from build123d import *

# Parameters (mm, degrees)
SKETCH_1_W           = 50
SKETCH_1_H           = 50
EXTRUDE_1_DEPTH      = 10
SKETCH_6_R           = 10.1
CUT_EXTRUDE_4_DEPTH  = 2
SKETCH_7_R           = 5
CUT_EXTRUDE_5_DEPTH  = 72.161787499
SKETCH_10_R          = 1
CUT_EXTRUDE_6_DEPTH  = 2
SKETCH_11_R          = 1.25
CUT_EXTRUDE_7_DEPTH  = 8
SKETCH_12_R          = 1.4
CUT_EXTRUDE_8_DEPTH  = 5
FILLET_1_R           = 0.5
SKETCH_13_R          = 1.25
CUT_EXTRUDE_9_DEPTH  = 5
SKETCH_14_R          = 1.25
CUT_EXTRUDE_11_DEPTH = 6
CUT_EXTRUDE_START    = -6
SKETCH_15_R          = 1.25
CUT_EXTRUDE_12_DEPTH = 6
SKETCH_16_R          = 1.25
CUT_EXTRUDE_13_DEPTH = 6
SKETCH_17_R          = 1.25
CUT_EXTRUDE_14_DEPTH = 6


with BuildPart() as part:
    # 草图1 → 凸台-拉伸1 (new body)
    with BuildSketch(Plane(origin=(0, 0, 0), x_dir=(1, 0, 0), z_dir=(0, 1, 0))):
        with Locations((25, 25)):
            Rectangle(SKETCH_1_W, SKETCH_1_H)
    extrude(amount=EXTRUDE_1_DEPTH)

    # 草图6 → 切除-拉伸4 (cut)
    with BuildSketch(Plane(origin=(0, 0, 0), x_dir=(-1, 0, 0), z_dir=(0, -1, 0))):
        with Locations(Location((-25, 11.5, 0), (0, 0, 90))):
            Circle(SKETCH_6_R)
    extrude(amount=-CUT_EXTRUDE_4_DEPTH, mode=Mode.SUBTRACT)

    # 草图7 → 切除-拉伸5 (cut, through all)
    with BuildSketch(Plane(origin=(0, 2, 0), x_dir=(-1, 0, 0), z_dir=(0, -1, 0))):
        with Locations(Location((-25, 11.5, 0), (0, 0, 90))):
            Circle(SKETCH_7_R)
    extrude(amount=-CUT_EXTRUDE_5_DEPTH, mode=Mode.SUBTRACT)

    # 草图10 → 切除-拉伸6 (cut)
    with BuildSketch(Plane(origin=(0, 10, 0), x_dir=(1, 0, 0), z_dir=(0, 1, 0))):
        with Locations(Location((25, 39, 0), (0, 0, 270))):
            Circle(SKETCH_10_R)
        with Locations(Location((11, 11, 0), (0, 0, 270))):
            Circle(SKETCH_10_R)
        with Locations(Location((39, 11, 0), (0, 0, 270))):
            Circle(SKETCH_10_R)
    extrude(amount=-CUT_EXTRUDE_6_DEPTH, mode=Mode.SUBTRACT)

    # 草图11 → 切除-拉伸7 (cut)
    with BuildSketch(Plane(origin=(0, 0, 0), x_dir=(-1, 0, 0), z_dir=(0, -1, 0))):
        with Locations(Location((-40, 18.4, 0), (0, 0, 90))):
            Circle(SKETCH_11_R)
        with Locations(Location((-40, 4.6, 0), (0, 0, 90))):
            Circle(SKETCH_11_R)
        with Locations(Location((-10, 18.4, 0), (0, 0, 90))):
            Circle(SKETCH_11_R)
        with Locations(Location((-10, 4.6, 0), (0, 0, 90))):
            Circle(SKETCH_11_R)
    extrude(amount=-CUT_EXTRUDE_7_DEPTH, mode=Mode.SUBTRACT)

    # 草图12 → 切除-拉伸8 (cut)
    with BuildSketch(Plane(origin=(0, 10, 0), x_dir=(1, 0, 0), z_dir=(0, 1, 0))):
        with Locations(Location((15, 29, 0), (0, 0, 270))):
            Circle(SKETCH_12_R)
        with Locations(Location((5, 29, 0), (0, 0, 270))):
            Circle(SKETCH_12_R)
        with Locations(Location((15, 46, 0), (0, 0, 270))):
            Circle(SKETCH_12_R)
        with Locations(Location((5, 46, 0), (0, 0, 270))):
            Circle(SKETCH_12_R)
    extrude(amount=-CUT_EXTRUDE_8_DEPTH, mode=Mode.SUBTRACT)

    # 圆角1
    fillet_1_edges = [part.edges().sort_by_distance(p)[0] for p in [
        (25, 10, -40),
        (11, 10, -12),
        (39, 10, -12),
    ]]
    fillet(fillet_1_edges, radius=FILLET_1_R)

    # 草图13 → 切除-拉伸9 (cut)
    with BuildSketch(Plane(origin=(0, 0, 0), x_dir=(-1, 0, 0), z_dir=(0, -1, 0))):
        with Locations(Location((-17.5, 29, 0), (0, 0, 90))):
            Circle(SKETCH_13_R)
        with Locations(Location((-32.5, 29, 0), (0, 0, 90))):
            Circle(SKETCH_13_R)
        with Locations(Location((-17.5, 45, 0), (0, 0, 90))):
            Circle(SKETCH_13_R)
        with Locations(Location((-32.5, 45, 0), (0, 0, 90))):
            Circle(SKETCH_13_R)
    extrude(amount=-CUT_EXTRUDE_9_DEPTH, mode=Mode.SUBTRACT)

    # 草图14 → 切除-拉伸11 (cut)
    with BuildSketch(Plane.ZY):
        with Locations((-25.000214672, 5)):
            Circle(SKETCH_14_R)
    extrude(amount=-CUT_EXTRUDE_11_DEPTH, mode=Mode.SUBTRACT)

    # 草图15 → 切除-拉伸12 (cut)
    with BuildSketch(Plane(origin=(50, 0, 0), x_dir=(0, 0, -1), z_dir=(1, 0, 0)).offset(CUT_EXTRUDE_START)):
        with Locations(Location((25.000214672, 5, 0), (0, 0, 180))):
            Circle(SKETCH_15_R)
    extrude(amount=CUT_EXTRUDE_12_DEPTH, mode=Mode.SUBTRACT)

    # 草图16 → 切除-拉伸13 (cut)
    with BuildSketch(Plane(origin=(0, 0, -50), x_dir=(-1, 0, 0), z_dir=(0, 0, -1))):
        with Locations((-25, 5)):
            Circle(SKETCH_16_R)
    extrude(amount=-CUT_EXTRUDE_13_DEPTH, mode=Mode.SUBTRACT)

    # 草图17 → 切除-拉伸14 (cut)
    with BuildSketch(Plane.XY.offset(CUT_EXTRUDE_START)):
        with Locations(Location((25, 5, 0), (0, 0, 180))):
            Circle(SKETCH_17_R)
    extrude(amount=CUT_EXTRUDE_14_DEPTH, mode=Mode.SUBTRACT)


solid = part.part
Could you check a few things on this model? Use its own coordinates, in mm. A direction names the side the tool comes from. Give positions to 0.01 mm unless a question says otherwise; leave off trailing zeros. Loops run counter-clockwise (first coordinate to the right, second up) from the corner with the lowest first, then second, coordinate; pieces in that order, holes last. Notation, with made-up numbers: M -8.5,59 L -1.5,59 A10 ccw -1.5,66 Z; hole C 19,32 d1. An arc over 180 degrees is marked long. Answer as a JSON object with one key per item and string values.
Q1. Suppose I cut it at A-A, the plane y = 1. State how many separate pieces and enclosed holes the cut face has, plus the area to 3 significant figures.
Values found:
{"separate pieces": "1", "enclosed holes": "9", "area": "2,140 mm²"}
Q2. Suppose I cut it at C-C, the plane z = -11. List the corners of the cut face in (x, y) for me.
Values found:
{"outline": "M 0,0 L 14.91,0 L 14.91,2 L 20.03,2 L 20.03,10 L 12.5,10 A0.5 ccw 12,9.5 L 12,8 L 10,8 L 10,9.5 A0.5 ccw 9.5,10 L 0,10 Z; M 29.97,2 L 35.09,2 L 35.09,0 L 50,0 L 50,10 L 40.5,10 A0.5 ccw 40,9.5 L 40,8 L 38,8 L 38,9.5 A0.5 ccw 37.5,10 L 29.97,10 Z"}
Q3. For faces 4 (the cylindrical face through (23.845, 5.479, -3.042)), 5 (the flat face through (10, 8, -18)), 6 (the flat face through (15, 5, -46)), which set-ups out of +Z, -Z, +X, -X, +Y, -Y let a thin tool reach every point of the face, with its end or its side?
Values found:
{"face 4": "+Z", "face 5": "-Y", "face 6": "+Y"}
Q4. If I drill on probe 1 along X at (y, z) = (3, -45); probe 2 along X at (y, z) = (6.75, -18.4); probe 3 along X at (y, z) = (1.75, -18.5), over which ranges is the centre line in solid material (lowest first)? Write a range as [from, to].
Values found:
{"probe 1": "x = [0, 16.25], [18.75, 31.25], [33.75, 50]", "probe 2": "x = [0, 8.75], [11.25, 38.75], [41.25, 50]", "probe 3": "x = [0, 8.75], [11.25, 17.72], [32.28, 38.75], [41.25, 50]"}
Q5. For P1, Ø2, axis at x = 40, z = -4.6, coming from the -Y side; P2, Ø0.8, axis at x = 4.5, z = -46.5, coming from the +Y side; P3, Ø1.6, axis at x = 11, z = -11.5, coming from the +Y side, each with a flat end and sliding along its axis, tell me the tip position at first contact or that it passes through.
Values found:
{"P1": "stops at y = 8", "P2": "stops at y = 5", "P3": "stops at y = 9.96"}
Q6. If we mould it in two halves opening along Z, with no side actions, what happens to faces 1 (the cylindrical face through (23.845, 4.521, -47.042)), 2 (the cylindrical face through (15.95, 7.54, -30.03)), 3 (the flat face through (25, 5, -6))? For each: pulls with the +Z half, pulls with the -Z half, needs draft (parallel to the pull), parting line crosses it, or undercut.
Values found:
{"face 1": "needs draft", "face 2": "undercut", "face 3": "pulls with the +Z half"}
Q7. Suppose I cut it at B-B, the plane x = 29. List the corners of the cut face in (y, z) for me, plus the area to 3 significant figures.
Values found:
{"outline": "M 0,-50 L 10,-50 L 10,-14.5 L 2,-14.5 L 2,-20.77 L 0,-20.77 Z; M 0,-2.23 L 2,-2.23 L 2,-8.5 L 10,-8.5 L 10,0 L 0,0 Z", "area": "415 mm²"}
Q8. Suppose I cut it at D-D, the plane z = -21. List the corners of the cut face in (x, y) for me.
Values found:
{"outline": "M 0,0 L 21.57,0 L 21.57,2 L 28.43,2 L 28.43,0 L 50,0 L 50,10 L 0,10 Z"}
